```python
from build123d import *

# Parameters (mm, degrees)
BOSS_EXTRUDE6_DEPTH     = 2.25
BOSS_EXTRUDE6_2_DEPTH   = 2.25
BOSS_EXTRUDE7_DEPTH     = 10
BOSS_EXTRUDE8_START     = -2.5
BOSS_EXTRUDE8_DEPTH     = 2.5
SKETCH8_R               = 0.5
CUT_EXTRUDE1_DEPTH      = 1
CUT_EXTRUDE1_DEPTH_BACK = 11


with BuildPart() as part:
    # Sketch7 → Boss-Extrude6 (new body)
    with BuildSketch(Plane.XY):
        with BuildLine():
            Line((28.537398615, 16.333832112), (-22.352574149, 16.333832112))
            Line((-22.352574149, 16.333832112), (-19.910011337, 10.634068342))
            ThreePointArc((-19.910011337, 10.634068342), (-19.816511792, 10.522258081), (-19.67689491, 10.480415214))
            Line((-19.67689491, 10.480415214), (25.816632323, 10.480415214))
            ThreePointArc((25.816632323, 10.480415214), (25.943590008, 10.484966358), (26.052322057, 10.550664975))
            Line((26.052322057, 10.550664975), (28.537398615, 16.333832112))
        make_face()
    extrude(amount=-BOSS_EXTRUDE6_DEPTH)



with BuildPart() as body_2:
    # Sketch7 → Boss-Extrude6 2 (new body)
    with BuildSketch(Plane.XY):
        with BuildLine():
            Line((113.387398615, 16.333832112), (62.497425851, 16.333832112))
            Line((62.497425851, 16.333832112), (64.939988663, 10.634068342))
            ThreePointArc((64.939988663, 10.634068342), (65.033488208, 10.522258081), (65.17310509, 10.480415214))
            Line((65.17310509, 10.480415214), (110.666632323, 10.480415214))
            ThreePointArc((110.666632323, 10.480415214), (110.793590008, 10.484966358), (110.902322057, 10.550664975))
            Line((110.902322057, 10.550664975), (113.387398615, 16.333832112))
        make_face()
    extrude(amount=-BOSS_EXTRUDE6_2_DEPTH)


with BuildPart() as part_1:
    add(part.part)

    add(body_2.part)  # Boss-Extrude7 merges body 2
    # Sketch7<12> → Boss-Extrude7 (add)
    with BuildSketch(Plane.XY):
        Polygon((130.21331835, 21.333832112), (130.21331835, 16.333832112), (125.46156201, 16.333832112), (113.387398615, 16.333832112), (62.497425851, 16.333832112), (50.366516028, 16.333832112), (40.61156201, 16.333832112), (28.537398615, 16.333832112), (-22.352574149, 16.333832112), (-34.483483972, 16.333832112), (-39.23668165, 16.333832112), (-39.23668165, 21.333832112), align=None)
    extrude(amount=-BOSS_EXTRUDE7_DEPTH)

    # Sketch7<13> → Boss-Extrude8 (add)
    with BuildSketch(Plane.XY.offset(BOSS_EXTRUDE8_START)):
        with BuildLine():
            Line((-34.736999841, 8.480030179), (-39.23668165, 8.480030179))
            Line((-39.23668165, 8.480030179), (-39.23668165, 16.333832112))
            Line((-39.23668165, 16.333832112), (-34.483483972, 16.333832112))
            Line((-34.483483972, 16.333832112), (-34.483483972, 8.733645436))
            ThreePointArc((-34.483483972, 8.733645436), (-34.557731024, 8.554347504), (-34.736999841, 8.480030179))
        make_face()
        with BuildLine():
            Line((40.61156201, 8.615866414), (40.61156201, 16.333832112))
            Line((40.61156201, 16.333832112), (50.366516028, 16.333832112))
            Line((50.366516028, 16.333832112), (50.366516028, 8.61586641))
            ThreePointArc((50.366516028, 8.61586641), (50.292268976, 8.436568478), (50.113000159, 8.362251153))
            Line((50.113000159, 8.362251153), (40.86508696, 8.362251153))
            ThreePointArc((40.86508696, 8.362251153), (40.685812272, 8.43656527), (40.61156201, 8.615866414))
        make_face()
        with BuildLine():
            Line((125.46156201, 8.615866414), (125.46156201, 16.333832112))
            Line((125.46156201, 16.333832112), (130.21331835, 16.333832112))
            Line((130.21331835, 16.333832112), (130.21331835, 8.362251153))
            Line((130.21331835, 8.362251153), (125.71508696, 8.362251153))
            ThreePointArc((125.71508696, 8.362251153), (125.535812272, 8.43656527), (125.46156201, 8.615866414))
        make_face()
    extrude(amount=-BOSS_EXTRUDE8_DEPTH)

    # Sketch8 → Cut-Extrude1 (cut, two sides)
    with BuildSketch(Plane.XY) as cut_extrude1_sk:
        with Locations((-36.73668165, 11.983669629)):
            Circle(SKETCH8_R)
        with Locations((-15.856255457, 13.233669629)):
            Circle(SKETCH8_R)
        with Locations((22.035256017, 13.233669629)):
            Circle(SKETCH8_R)
        with Locations((42.86331835, 11.983669629)):
            Circle(SKETCH8_R)
        with Locations((48.11331835, 11.983669629)):
            Circle(SKETCH8_R)
        with Locations((68.993744543, 13.233669629)):
            Circle(SKETCH8_R)
        with Locations((106.885256017, 13.233669629)):
            Circle(SKETCH8_R)
        with Locations((127.71331835, 11.983669629)):
            Circle(SKETCH8_R)
    extrude(amount=CUT_EXTRUDE1_DEPTH, mode=Mode.SUBTRACT)
    extrude(cut_extrude1_sk.sketch, amount=-CUT_EXTRUDE1_DEPTH_BACK, mode=Mode.SUBTRACT)


solid = part_1.part
```
Geometry check sheet. Reference: the model listing, model coordinates, mm. A direction names the side the tool comes from. Round coordinates to 2 decimals unless told otherwise and drop trailing zeros. Loops run counter-clockwise (first coordinate to the right, second up) from the corner with the lowest first, then second, coordinate; pieces in that order, holes last. Notation, with made-up numbers: (39, 77) - (45, 77) arc R31 ccw to (45, 112) - close; hole circle Ø5 at (43.25, 41.25). An arc over 180 degrees is marked (long way). Use a Markdown table: item, result.
Q1. Cross-section at B-B on z = -6.5. Record the cut outline in (x, y), plus the area to 3 significant figures.
Solutions:
| item | result |
|---|---|
| outline | (-39.24, 16.33) - (130.21, 16.33) - (130.21, 21.33) - (-39.24, 21.33) - close |
| area | 847 mm2 |
Q2. Material ranges on line 1 (X direction, y = 10, z = -2.75); line 2 (Y direction, x = 7.5, z = -7.25); line 3 (Z direction, x = 108, y = 11.5), recorded low to high.
Solutions:
| item | result |
|---|---|
| line 1 | x = -39.24 to -34.48, 40.61 to 50.37, 125.46 to 130.21 |
| line 2 | y = 16.33 to 21.33 |
| line 3 | z = -2.25 to 0 |
Q3. Draft check along X on faces 1 (the flat face through (-39.237, 16, -4)), 2 (the flat face through (47, 17, 0)), 3 (the flat face through (44, 16.334, -6)), 4 (the flat face through (130.213, 16, -4)). Enter one of: released by +X, released by -X, zero draft, split by the parting line, or undercut.
Solutions:
| item | result |
|---|---|
| face 1 | released by -X |
| face 2 | zero draft |
| face 3 | undercut |
| face 4 | released by +X |
Q4. Cross-section at A-A on x = 17. Record the cut outline in (y, z).
Solutions:
| item | result |
|---|---|
| outline | (10.48, -2.25) - (16.33, -2.25) - (16.33, -10) - (21.33, -10) - (21.33, 0) - (10.48, 0) - close |
Q5. Go/stop test with flat-tipped pins: P1, Ø4, axis at x = -36.5, y = 11.5, coming from the -Z side; P2, Ø1.4, axis at x = 127, y = 10.5, coming from the +Z side; P3, Ø5, axis at x = 27.5, z = -2, coming from the -Y side. Record where each tip stops, or that it passes through.
Solutions:
| item | result |
|---|---|
| P1 | stops at z = -5 |
| P2 | stops at z = -2.5 |
| P3 | stops at y = 10.47 |
Q6. Cross-section at C-C on x = 56.5. Record the cut outline in (y, z).
Solutions:
| item | result |
|---|---|
| outline | (16.33, -10) - (21.33, -10) - (21.33, 0) - (16.33, 0) - close |
Q7. Access from +Z, -Z, +X, -X, +Y, -Y to the whole of each face (thin tool, end or side, straight path). Record for faces 5 (the flat face through (127, 12, -5)), 6 (the flat face through (-36, 12, -2.5)), 7 (the flat face through (47, 19, -10)).
Solutions:
| item | result |
|---|---|
| face 5 | -Z, +X, -X, -Y |
| face 6 | +Z, +X, -X, -Y |
| face 7 | -Z, +X, -X, +Y, -Y |
